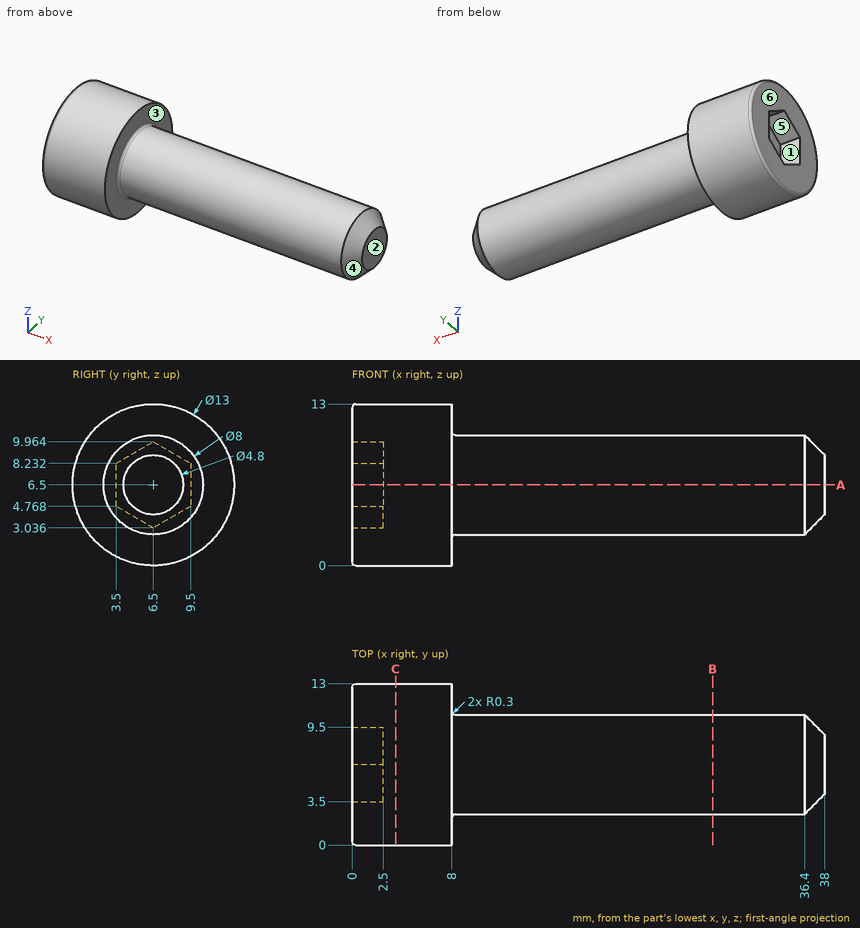
Could you check a few things on this drawing? It's one solid part, dimensions in mm from its lowest x, y, z. A direction names the side the tool comes from. Coordinates: 2 decimals unless noted, no trailing zeros. Write each loop counter-clockwise with the first axis right and the second up, starting at its lowest first coordinate (ties: lowest second). Pieces come first, ordered by that corner, then holes. Notation, with made-up numbers: (0.5, 0) - (29.5, 0) arc R22 cw to (29.5, 24) - close; hole circle Ø8 at (20, 88.25). An arc over 180 degrees is marked (long way). Use one line per item in the form item = value.
1) On a 3-axis mill with a long thin cutter (end or side, diameter ignored), from which of +Z, -Z, +X, -X, +Y, -Y can I reach the whole of each face in a straight line? I mean the marked faces 1, 2 and 3. Say none if no direction works.
Solved:
face_1 = -X
face_2 = +Z, -Z, +X, +Y, -Y
face_3 = +X
2) Suppose I cut it at B-B, the plane x = 29. Write out the boundary of the cut face in (y, z), plus the area to 3 significant figures.
Solved:
outline = circle Ø8 at (6.5, 6.5)
area = 50.3 mm2
3) Suppose I cut it at A-A, the plane z = 6.5. Write out the boundary of the cut face in (x, y), plus the area to 3 significant figures.
Solved:
outline = (0, 0.3) arc R0.3 ccw to (0.3, 0) - (8, 0) - (8, 2.2) arc R0.3 cw to (8.3, 2.5) - (36.4, 2.5) - (38, 4.1) - (38, 8.9) - (36.4, 10.5) - (8.3, 10.5) arc R0.3 cw to (8, 10.8) - (8, 13) - (0.3, 13) arc R0.3 ccw to (0, 12.7) - (0, 9.5) - (2.5, 9.5) - (2.5, 3.5) - (0, 3.5) - close
area = 326 mm2
4) I need wall thicknesses on line 1 (Z direction, x = 12.5, y = 4.5); line 2 (X direction, y = 10, z = 3.5); line 3 (X direction, y = 5.5, z = 5.75). Which ranges of each line are inside material? Lowest first, please.
Solved:
line_1 = 3.04 to 9.96
line_2 = 0 to 8
line_3 = 2.5 to 38
5) Suppose I cut it at C-C, the plane x = 3.5. Write out the boundary of the cut face in (y, z), plus the area to 3 significant figures.
Solved:
outline = circle Ø13 at (6.5, 6.5)
area = 133 mm2
6) I'm going to push flat-ended pins straight in: P1, Ø1, axis at y = 2.5, z = 8.5, coming from the -X side; P2, Ø1, axis at x = 5, y = 11.5, coming from the +Z side; P3, Ø1.5, axis at x = 17, z = 8.5, coming from the +Y side; P4, Ø6, axis at x = 26.5, z = 5.5, coming from the +Y side. Where does each tip first touch, or does it pass through?
Solved:
P1 = 0
P2 = 11.19
P3 = 10.3
P4 = 10.5
7) Thinking about a two-plate mould opening in Z: for the marked faces 4, 5 and 6, which applies, released by +Z, released by -Z, zero draft, split by the parting line, or undercut?
Solved:
face_4 = split by the parting line
face_5 = undercut
face_6 = zero draft
